The figure shows three views and two pictorial views of one solid part (mm, origin at its lowest corner). Answer the questions. A direction names the side the tool comes from. Round coordinates to 2 decimals unless told otherwise and drop trailing zeros. Order: outer loops, then holes, each group sorted by start corner. A loop starts at its lowest first (then second) coordinate and runs counter-clockwise, first axis right, second up.
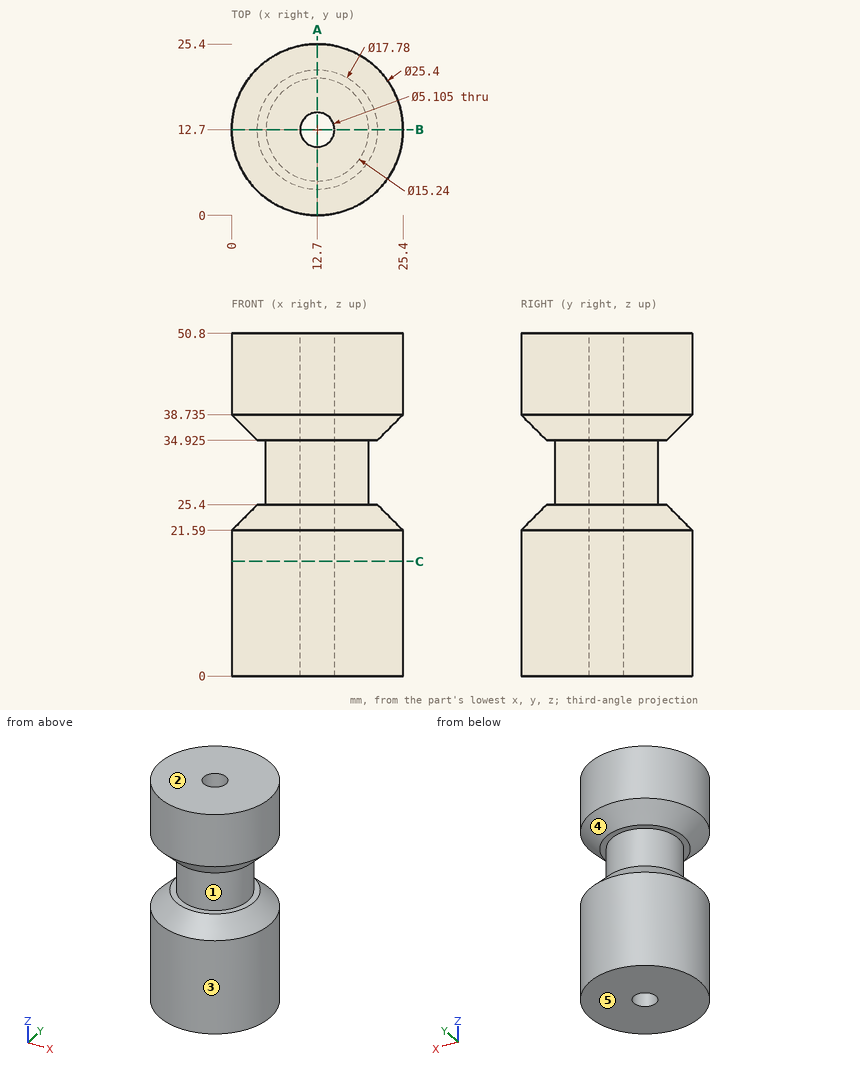
Item 1: Find section A-A (x = 12.7). Write down the section's boundary in (y, z) (1 decimal), plus the area to 3 significant figures.
Item 2: Find the intervals of material crossed by line 1 along X through (y, z) = (12.7, 18); line 2 along X through (y, z) = (12.7, 32); line 3 along Z through (x, y) = (5.25, 8) (1 decimal), in increasing order.
Item 3: Given pin 1 (4 mm diameter, centred on x = 12.7, y = 12.7, fed in from -Z); pin 2 (2 mm diameter, centred on x = 9, z = 40, fed in from -Y); pin 3 (1 mm diameter, centred on y = 2.5, z = 37.5, fed in from +X); pin 4 (12 mm diameter, centred on x = 4, z = 7.5, fed in from +Y), each flat-ended and moving along its own axis, determine where each tip first touches the part or whether it passes through.
Item 4: Find section C-C (z = 17). Write down the section's boundary in (x, y) (1 decimal), plus the area to 3 significant figures.
Item 5: A tool of negligible diameter and unlimited length cuts with its end or side. For the marked faces 4 and 5, from which of +Z, -Z, +X, -X, +Y, -Y can it reach the whole face along a straight path? Write none if from no direction.
Item 6: For a pull along Z with two mould halves and no side action, classify the marked faces 1, 2 and 3 as released by +Z, released by -Z, zero draft, split by the parting line, or undercut.
Model answer:
1. outline: (0, 0) - (10.1, 0) - (10.1, 50.8) - (0, 50.8) - (0, 38.7) - (3.8, 34.9) - (5.1, 34.9) - (5.1, 25.4) - (3.8, 25.4) - (0, 21.6) - close; (15.3, 0) - (25.4, 0) - (25.4, 21.6) - (21.6, 25.4) - (20.3, 25.4) - (20.3, 34.9) - (21.6, 34.9) - (25.4, 38.7) - (25.4, 50.8) - (15.3, 50.8) - close
1. area: 905 mm2
2. line 1: x = 0 to 10.15, 15.25 to 25.4
2. line 2: x = 5.08 to 10.15, 15.25 to 20.32
2. line 3: z = 0 to 25.4, 34.9 to 50.8
3. pin 1: passes through
3. pin 2: stops at y = 0.29
3. pin 3: stops at x = 19.24
3. pin 4: stops at y = 25.11
4. outline: circle Ø25.4 at (12.7, 12.7); hole circle Ø5.1 at (12.7, 12.7)
4. area: 486 mm2
5. face 4: none
5. face 5: -Z, +X, -X, +Y, -Y
6. face 1: undercut
6. face 2: released by +Z
6. face 3: zero draft
